Can you work these out from the model? Positions are in its coordinate system, mm. Face numbers are marked on the shaded views. A direction names the side the tool comes from. Round coordinates to 2 decimals unless told otherwise and drop trailing zeros. Loops run counter-clockwise (first coordinate to the right, second up) from the corner with the lowest first, then second, coordinate; pieces in that order, holes last. Notation, with made-up numbers: M -33,-26.75 L -10,-26.75 A18 ccw -10,-18.75 Z; hole C 17.5,64 d2. An arc over 180 degrees is marked long. Return JSON: item names as keys, results as strings.
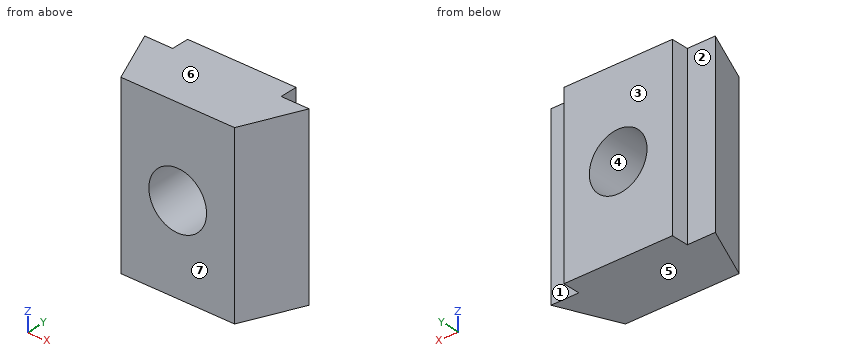
```python
from build123d import *

# Parameters (mm, degrees)
BOSS_EXTRUDE1_DEPTH       = 5
M4X0_7_TAPPED_HOLE2_D     = 3.3
M4X0_7_TAPPED_HOLE2_DEPTH = 11.5
M4X0_7_TAPPED_HOLE2_TIP   = 0.991420021


with BuildPart() as part:
    # Sketch1 → Boss-Extrude1 (new, symmetric)
    with BuildSketch(Plane.XY):
        Polygon((-3.25, 0), (3.25, 0), (4.7, 3.3), (3.1, 3.3), (3.1, 4.3), (-3.1, 4.3), (-3.1, 3.3), (-4.7, 3.3), align=None)
    extrude(amount=BOSS_EXTRUDE1_DEPTH, both=True)

    # M4x0.7 Tapped Hole2
    with Locations(Plane(origin=(0, 4.3, 0), x_dir=(1, 0, 0), z_dir=(0, 1, 0))):
        with Locations((0, 0)):
            Hole(M4X0_7_TAPPED_HOLE2_D / 2, depth=M4X0_7_TAPPED_HOLE2_DEPTH)
            with Locations((0, 0, -(M4X0_7_TAPPED_HOLE2_DEPTH + M4X0_7_TAPPED_HOLE2_TIP / 2))):  # 118° drill point
                Cone(0, M4X0_7_TAPPED_HOLE2_D / 2, M4X0_7_TAPPED_HOLE2_TIP, mode=Mode.SUBTRACT)


solid = part.part
```
Q1. Suppose I cut it at A-A, the plane z = 0. Please give me the cut outline in (x, y).
Results:
{"outline": "M -4.7,3.3 L -3.25,0 L -1.65,0 L -1.65,4.3 L -3.1,4.3 L -3.1,3.3 Z; M 1.65,0 L 3.25,0 L 4.7,3.3 L 3.1,3.3 L 3.1,4.3 L 1.65,4.3 Z"}
Q2. If I drill on line 1 along Z through (x, y) = (0, 1.6); line 2 along X through (y, z) = (3.6, 4.5); line 3 along X through (y, z) = (1.65, -1.25) (3 decimals), over which ranges is the centre line in solid material (lowest first)?
Results:
{"line 1": "z = -5 to -1.65, 1.65 to 5", "line 2": "x = -3.1 to 3.1", "line 3": "x = -3.975 to -1.077, 1.077 to 3.975"}
Q3. Suppose I cut it at D-D, the plane y = 3.15. Please give me the cut outline in (x, z), plus the area to 3 significant figures.
Results:
{"outline": "M -4.63,-5 L 4.63,-5 L 4.63,5 L -4.63,5 Z; hole C 0,0 d3.3", "area": "84.1 mm2"}
Q4. I'm going to push flat-ended pins straight in: pin 1 Ø0.5 at (x, z) = (-4, 0.5) entering from +Y; pin 2 Ø0.5 at (y, z) = (4, -1) entering from -X; pin 3 Ø2 at (x, z) = (0, 0) entering from +Y; pin 4 Ø1.1 at (y, z) = (4, 0.5) entering from +X. Where does each tip first touch, or does it pass through?
Results:
{"pin 1": "stops at y = 3.3", "pin 2": "stops at x = -3.1", "pin 3": "passes through", "pin 4": "stops at x = 3.1"}
Q5. Suppose I cut it at C-C, the plane z = -4. Please give me the cut outline in (x, y), plus the area to 3 significant figures.
Results:
{"outline": "M -4.7,3.3 L -3.25,0 L 3.25,0 L 4.7,3.3 L 3.1,3.3 L 3.1,4.3 L -3.1,4.3 L -3.1,3.3 Z", "area": "32.4 mm2"}
Q6. Thinking about a two-plate mould opening in Z: for the marked faces 4, 5, 6 and 7, which applies, pulls with the +Z half, pulls with the -Z half, needs draft (parallel to the pull), parting line crosses it, or undercut?
Results:
{"face 4": "undercut", "face 5": "pulls with the -Z half", "face 6": "pulls with the +Z half", "face 7": "needs draft"}
Q7. Suppose I cut it at B-B, the plane x = 0. Please give me the cut outline in (y, z), plus the area to 3 significant figures.
Results:
{"outline": "M 0,-5 L 4.3,-5 L 4.3,-1.65 L 0,-1.65 Z; M 0,1.65 L 4.3,1.65 L 4.3,5 L 0,5 Z", "area": "28.8 mm2"}
Q8. On a 3-axis mill with a long thin cutter (end or side, diameter ignored), from which of +Z, -Z, +X, -X, +Y, -Y can I reach the whole of each face in a straight line? I mean the marked faces 1, 2 and 3. Say none if no direction works.
Results:
{"face 1": "+Z, -Z, +X, +Y", "face 2": "+Z, -Z, -X, +Y", "face 3": "+Z, -Z, +X, -X, +Y"}
